Verification items for the finished model (mm, model axes). Face numbers are marked on the shaded views. Coordinates: 2 decimals unless noted, no trailing zeros. Order: outer loops, then holes, each group sorted by start corner. A loop starts at its lowest first (then second) coordinate and runs counter-clockwise, first axis right, second up. Notation, with made-up numbers: M -26.5,65.5 L 16.5,65.5 A18 cw 16.5,90.5 Z; hole C 82.5,-24.75 d10. An arc over 180 degrees is marked long. Return JSON: item names as keys, results as strings. Group by question number.
Q1. Thickness scan on probe 1 along Z at (x, y) = (-0.5, -6.5); probe 2 along Z at (x, y) = (-41.5, -11.75); probe 3 along X at (y, z) = (-6, 11). Record the ranges inside material, lowest first.
Q2. Section check D-D, the plane z = -193. Enter the section's corners in (x, y).
Q3. Mould release check, pull along Z, two halves, no side actions. Record for the marked faces 1 and 2: pulls with the +Z half, pulls with the -Z half, needs draft (parallel to the pull), parting line crosses it, or undercut.
Q4. Section check A-A, the plane y = -14.75. Enter the section's corners in (x, z).
Q5. Section check C-C, the plane x = 81. Enter the section's corners in (y, z), then the cut area to 3 significant figures.
Q6. Section check B-B, the plane z = -4. Enter the section's corners in (x, y).
Q7. Go/stop test with a flat-tipped pin: pin 1 Ø14 at (x, z) = (-46.5, 99) entering from -Y. Record where the tip stops, or that it passes through.
from build123d import *

# Parameters (mm, degrees)
F0_W      = 300
F0_H      = 400
F1_DEPTH  = 19
F2_W      = 279
F2_H      = 46
F3_DEPTH  = 10
F4_W      = 140
F4_H      = 10
F5_DEPTH  = 10
F6_W      = 260
F6_H      = 312
F7_DEPTH  = 19
F8_W      = 10
F8_H      = 80
F9_DEPTH  = 19
F10_W     = 10
F10_H     = 80
F11_DEPTH = 19


with BuildPart() as f1:
    # F0 (on Front) → F1 (new body)
    with BuildSketch(Plane.XZ):
        with Locations((5.324256, -69.15618)):
            Rectangle(F0_W, F0_H)
    extrude(amount=F1_DEPTH)

    # F2 (on face) → F3 (cut)
    with BuildSketch(Plane.XZ.offset(19)):
        with Locations((5.324256, 97.84382)):
            Rectangle(F2_W, F2_H)
    extrude(amount=-F3_DEPTH, mode=Mode.SUBTRACT)

    # F4 (on face) → F5 (cut)
    with BuildSketch(Plane.XZ.offset(9)):
        with Locations((5.324256, 79.84382)):
            Rectangle(F4_W, F4_H)
    extrude(amount=-F5_DEPTH, mode=Mode.SUBTRACT)

    # F6 (on face) → F7 (cut)
    with BuildSketch(Plane.XZ.offset(19)):
        with Locations((5.324256, -91.15618)):
            Rectangle(F6_W, F6_H)
    extrude(amount=-F7_DEPTH, mode=Mode.SUBTRACT)

    # F8 (on face) → F9 (cut)
    with BuildSketch(Plane(origin=(0, 0, 0), x_dir=(-1, 0, 0), z_dir=(0, 1, 0))):
        with Locations((-140.324256, -199.15618)):
            Rectangle(F8_W, F8_H)
    extrude(amount=-F9_DEPTH, mode=Mode.SUBTRACT)

    # F10 (on face) → F11 (cut)
    with BuildSketch(Plane(origin=(0, 0, 0), x_dir=(-1, 0, 0), z_dir=(0, 1, 0))):
        with Locations((129.675744, -199.15618)):
            Rectangle(F10_W, F10_H)
    extrude(amount=-F11_DEPTH, mode=Mode.SUBTRACT)


solid = f1.part
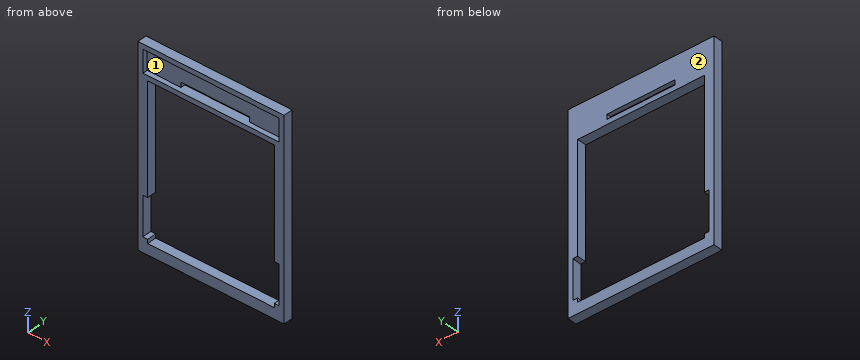
Numbers:
{
 "1": {"probe 1": "z = -269.16 to -247.16, 64.84 to 74.84, 84.84 to 130.84", "probe 2": "z = -269.16 to -247.16, 64.84 to 74.84, 120.84 to 130.84", "probe 3": "x = -144.68 to -124.68, 135.32 to 155.32"},
 "2": {"outline": "M -144.68,-19 L -134.68,-19 L -134.68,0 L -144.68,0 Z; M 145.32,-19 L 155.32,-19 L 155.32,0 L 145.32,0 Z"},
 "3": {"face 1": "undercut", "face 2": "needs draft"},
 "4": {"outline": "M -144.68,-269.16 L 155.32,-269.16 L 155.32,130.84 L -144.68,130.84 Z; hole M -134.68,-239.16 L -124.68,-239.16 L -124.68,-247.16 L 135.32,-247.16 L 135.32,-239.16 L 145.32,-239.16 L 145.32,-159.16 L 135.32,-159.16 L 135.32,64.84 L -124.68,64.84 L -124.68,-159.16 L -134.68,-159.16 Z; hole M -134.18,74.84 L 144.82,74.84 L 144.82,120.84 L -134.18,120.84 Z"},
 "5": {"outline": "M -19,-269.16 L 0,-269.16 L 0,-247.16 L -19,-247.16 Z; M -19,64.84 L 0,64.84 L 0,130.84 L -19,130.84 L -19,120.84 L -9,120.84 L -9,74.84 L -19,74.84 Z", "area": "1,210 mm2"},
 "6": {"outline": "M -144.68,-19 L -124.68,-19 L -124.68,0 L -144.68,0 Z; M 135.32,-19 L 155.32,-19 L 155.32,0 L 135.32,0 Z"},
 "7": {"pin 1": "stops at y = -9"}
}
